```python
from build123d import *

# Parameters (mm, degrees)
SKETCH_1_W          = 48
SKETCH_1_H          = 24
EXTRUDE_1_DEPTH     = 1.5
FILLET_1_R          = 2
CUT_EXTRUDE_1_REACH = 3.5
SKETCH_2_R          = 2
SKETCH_3_R          = 11.5
EXTRUDE_2_DEPTH     = 9


with BuildPart() as part:
    # 草图1 → 凸台-拉伸1 (new body)
    with BuildSketch(Plane(origin=(0, 0, 0), x_dir=(1, 0, 0), z_dir=(0, 1, 0))):
        Rectangle(SKETCH_1_W, SKETCH_1_H)
    extrude(amount=EXTRUDE_1_DEPTH)

    # 圆角1
    fillet_1_edges = [part.edges().sort_by_distance(p)[0] for p in [
        (-24, 0.75, -12),
        (24, 0.75, -12),
        (24, 0.75, 12),
        (-24, 0.75, 12),
    ]]
    fillet(fillet_1_edges, radius=FILLET_1_R)

    # 草图2 → 切除-拉伸1 (cut, up to next)
    with BuildSketch(Plane(origin=(0, 1.5, 0), x_dir=(1, 0, 0), z_dir=(0, 1, 0)), mode=Mode.PRIVATE) as cut_extrude_1_sk1:
        with Locations((8, 8)):
            Circle(SKETCH_2_R)
    cut_extrude_1_tool1 = extrude(cut_extrude_1_sk1.sketch, amount=-CUT_EXTRUDE_1_REACH, mode=Mode.PRIVATE) & part.part
    add(cut_extrude_1_tool1.solids().sort_by_distance((8, 1.5, -8))[0], mode=Mode.SUBTRACT)
    # 草图2 → 切除-拉伸1 (cut, up to next)
    with BuildSketch(Plane(origin=(0, 1.5, 0), x_dir=(1, 0, 0), z_dir=(0, 1, 0)), mode=Mode.PRIVATE) as cut_extrude_1_sk2:
        with Locations((8, -8)):
            Circle(SKETCH_2_R)
    cut_extrude_1_tool2 = extrude(cut_extrude_1_sk2.sketch, amount=-CUT_EXTRUDE_1_REACH, mode=Mode.PRIVATE) & part.part
    add(cut_extrude_1_tool2.solids().sort_by_distance((8, 1.5, 8))[0], mode=Mode.SUBTRACT)

    # 草图3 → 凸台-拉伸2 (add)
    with BuildSketch(Plane(origin=(0, 1.5, 0), x_dir=(1, 0, 0), z_dir=(0, 1, 0))):
        with Locations((-12, 0)):
            Circle(SKETCH_3_R)
    extrude(amount=EXTRUDE_2_DEPTH)


solid = part.part
```
Work out the finished part from the listing and answer in its coordinate system (mm). A direction names the side the tool comes from. Give positions to 0.01 mm unless a question says otherwise; leave off trailing zeros. Order: outer loops, then holes, each group sorted by start corner. A loop starts at its lowest first (then second) coordinate and runs counter-clockwise, first axis right, second up.
1. The mould has two halves that part along X. Classify faces 3 (the cylindrical face through (6.526, 0.76, -9.352)), 4 (the flat face through (0, 1, -12)), 5 (the cylindrical face through (-23.43, 0.76, -11.4)): released by +X, released by -X, zero draft, split by the parting line, or undercut.
Result sheet:
face 3: undercut
face 4: zero draft
face 5: released by -X
2. Section B-B, the plane z = -6.75 is taken. Determine the outline of the cut face in (x, y), and give its area (3 significant figures).
Result sheet:
outline: (-24, 0) - (6.44, 0) - (6.44, 1.5) - (-2.69, 1.5) - (-2.69, 10.5) - (-21.31, 10.5) - (-21.31, 1.5) - (-24, 1.5) - close; (9.56, 0) - (24, 0) - (24, 1.5) - (9.56, 1.5) - close
area: 235 mm2
3. For faces 1 (the cylindrical face through (-13.5, 5.9, -11.4)), 2 (the flat face through (-24, 1, 0)), determine the directions among +Z, -Z, +X, -X, +Y, -Y from which every point of the face is accessible in a straight line to the end or side of a thin tool.
Result sheet:
face 1: +Y
face 2: +Z, -Z, -X, +Y, -Y
4. Section D-D, the plane z = 0 is taken. Determine the outline of the cut face in (x, y), and give its area (3 significant figures).
Result sheet:
outline: (-24, 0) - (24, 0) - (24, 1.5) - (-0.5, 1.5) - (-0.5, 10.5) - (-23.5, 10.5) - (-23.5, 1.5) - (-24, 1.5) - close
area: 279 mm2
5. Straight lines are drawn through the part: L1, parallel to Z at x = 8, y = 0.45; L2, parallel to X at y = 1.2, z = 8; L3, parallel to Y at x = 15.5, z = 3.5. For each, find the intervals that lie inside material, in ascending order.
Result sheet:
L1: z = -12 to -10, -6 to 6, 10 to 12
L2: x = -24 to 6, 10 to 24
L3: y = 0 to 1.5
6. Each of these flat-tipped pins is pushed along its axis until it touches: P1, Ø4, axis at y = 5.5, z = -7.5, coming from the -X side; P2, Ø5, axis at x = 8, z = 8, coming from the +Y side; P3, Ø4, axis at y = 6, z = -1, coming from the -X side. Where does it stop, or does it pass through?
Result sheet:
P1: stops at x = -22.1
P2: stops at y = 1.5
P3: stops at x = -23.5
7. Section C-C, the plane y = 1 is taken. Determine the outline of the cut face in (x, z), and give its area (3 significant figures).
Result sheet:
outline: (-24, -10) arc R2 ccw to (-22, -12) - (22, -12) arc R2 ccw to (24, -10) - (24, 10) arc R2 ccw to (22, 12) - (-22, 12) arc R2 ccw to (-24, 10) - close; hole circle Ø4 at (8, -8); hole circle Ø4 at (8, 8)
area: 1,120 mm2
8. Section A-A, the plane x = 8 is taken. Determine the outline of the cut face in (y, z).
Result sheet:
outline: (0, -12) - (1.5, -12) - (1.5, -10) - (0, -10) - close; (0, -6) - (1.5, -6) - (1.5, 6) - (0, 6) - close; (0, 10) - (1.5, 10) - (1.5, 12) - (0, 12) - close
